```python
from build123d import *

# Parameters (mm, degrees)
F0_R     = 30
F1_DEPTH = 5
F2_R     = 9.55
F3_DEPTH = 5.5
F4_R     = 2.0590521715
F6_R     = 6.4
F7_DEPTH = 5.1


with BuildPart() as f1:
    # F0 (on Top) → F1 (new body)
    with BuildSketch(Plane.XY):
        Circle(F0_R)
    extrude(amount=F1_DEPTH)

    # F2 (on face) → F3 (cut)
    with BuildSketch(Plane.XY.offset(5)):
        Circle(F2_R)
    extrude(amount=-F3_DEPTH, mode=Mode.SUBTRACT)

    # F5: sweep along a path in F0
    with BuildLine(Plane.XY) as f5_path:
        CenterArc((0, 0), 30, 0, 360)
    # F4 (on Right) → F5 (sweep, cut)
    with BuildSketch(Plane.YZ):
        with Locations((30.0044678152, 2.5)):
            Circle(F4_R)
    sweep(path=f5_path.line, mode=Mode.SUBTRACT)

    # F6 (on face) → F7 (cut)
    with BuildSketch(Plane.XY.offset(5)):
        with Locations((-20.3089937568, 0)):
            Circle(F6_R)
    extrude(amount=-F7_DEPTH, mode=Mode.SUBTRACT)


solid = f1.part
```
Design review of the part built by this model. Coordinates are the model's own, in mm. Coordinates: 2 decimals unless noted, no trailing zeros. Order: outer loops, then holes, each group sorted by start corner. A loop starts at its lowest first (then second) coordinate and runs counter-clockwise, first axis right, second up.
1) Wall thickness on line 1 along Y through (x, z) = (0, 2.6); line 2 along Y through (x, z) = (-15.5, 1.8); line 3 along X through (y, z) = (-7.5, 4.65): over which ranges is each line inside the solid? List them lowest first.
2) Take a section at B-B, the plane x = 0. Give the boundary of the cut face in (y, z).
3) Clearance check with flat-ended pins moving along their axes: pin 1 (3 mm diameter, centred on y = -22.5, z = 4.5, fed in from +X); pin 2 (1 mm diameter, centred on x = 21, z = 2, fed in from -Y); pin 3 (1 mm diameter, centred on x = 22, z = 2.5, fed in from -Y). State where each tip first meets the part, or that it passes through.
4) Take a section at C-C, the plane z = 3.05. Give the boundary of the cut face in (x, y).
5) Take a section at A-A, the plane y = 0. Give the boundary of the cut face in (x, z), and give its area (3 significant figures).
6) Mouldability with a two-part tool opening along Y and no side actions: class faces 1 (the cylindrical face through (-7.58, -5.81, 2.54)), 2 (the flat face through (-7, 7, 5)), 3 (the cylindrical face through (-29.97, 1.32, 4.78)), 4 (the cylindrical face through (-14.397, -2.451, 2.535)) as +Y half, -Y half, draft (parallel to the pull), parting line (faces both ways), or undercut.
Returned:
1. line 1: y = -27.95 to -9.55, 9.55 to 27.95
1. line 2: y = -23.4 to -4.22, 4.22 to 23.4
1. line 3: x = -29.05 to -5.91, 5.91 to 29.05
2. outline: (-30, 0) - (-9.55, 0) - (-9.55, 5) - (-30, 5) - (-30, 4.56) arc R2.06 cw to (-30, 0.44) - close; (9.55, 0) - (30, 0) - (30, 0.44) arc R2.06 cw to (30, 4.56) - (30, 5) - (9.55, 5) - close
3. pin 1: stops at x = 21.42
3. pin 2: stops at y = -19.13
3. pin 3: stops at y = -17.85
4. outline: circle Ø56.04 at (0, 0); hole circle Ø12.8 at (-20.31, 0); hole circle Ø19.1 at (0, 0)
5. outline: (-30, 0) - (-26.71, 0) - (-26.71, 5) - (-30, 5) - (-30, 4.56) arc R2.06 cw to (-30, 0.44) - close; (-13.91, 0) - (-9.55, 0) - (-9.55, 5) - (-13.91, 5) - close; (9.55, 0) - (30, 0) - (30, 0.44) arc R2.06 cw to (30, 4.56) - (30, 5) - (9.55, 5) - close
5. area: 127 mm2
6. face 1: undercut
6. face 2: draft
6. face 3: parting line
6. face 4: undercut
